Part model, mm, in its own coordinate system. A direction names the side the tool comes from. Coordinates: 2 decimals unless noted, no trailing zeros. Loops run counter-clockwise (first coordinate to the right, second up) from the corner with the lowest first, then second, coordinate; pieces in that order, holes last. Notation, with made-up numbers: M -38,-1 L -13,-1 A18 ccw -13,10 Z; hole C -8,70.5 d9. An arc over 180 degrees is marked long. Answer as a JSON object with one key per item and string values. Group by question number.
1. Saw through at C-C on z = 59. Write the cut outline in (x, y), then the cut area to 3 significant figures.
2. 3-axis set-ups, long thin cutter, end or side, ignore diameter. For faces 1 (the face through (-2, 6, 0)), 2 (the face through (-1.73, -7.81, 241.57)), 3 (the face through (-4, 4, 497)): which of +Z, -Z, +X, -X, +Y, -Y reach the whole face in a straight line?
3. Drill centre lines: L1, parallel to Z at x = -4.25, y = 5.75; L2, parallel to Y at x = 1.25, z = 266.5; L3, parallel to Z at x = 3.5, y = 3.5. Where is each one in solid material? Low to high.
4. Drop flat-ended pins along their axis: pin 1 Ø1 at (x, z) = (2.5, 115) entering from +Y; pin 2 Ø1 at (x, z) = (4, 143.5) entering from +Y; pin 3 Ø5 at (y, z) = (-5, 69) entering from +X. Give the stop position or say it passes through.
from build123d import *

# Parameters (mm, degrees)
SKETCH1_R           = 8
BOSS_EXTRUDE1_DEPTH = 490
SKETCH6_R           = 6
BOSS_EXTRUDE2_DEPTH = 5
SKETCH7_R           = 6
BOSS_EXTRUDE3_DEPTH = 2
SKETCH8_R           = 5
BOSS_EXTRUDE4_DEPTH = 10
SKETCH9_R           = 4
BOSS_EXTRUDE5_DEPTH = 10
CHAMFER1_SIZE       = 1
CHAMFER2_SIZE       = 1
BOSS_EXTRUDE6_START = 5
SKETCH10_R          = 6
BOSS_EXTRUDE6_DEPTH = 5
BOSS_EXTRUDE7_START = 2
SKETCH11_R          = 6
BOSS_EXTRUDE7_DEPTH = 2
BOSS_EXTRUDE8_START = 10
SKETCH12_R          = 5
BOSS_EXTRUDE8_DEPTH = 10
CHAMFER3_SIZE       = 1


with BuildPart() as part:
    # Sketch1 → Boss-Extrude1 (new body)
    with BuildSketch(Plane.XY):
        Circle(SKETCH1_R)
    extrude(amount=BOSS_EXTRUDE1_DEPTH)

    # Sketch6 → Boss-Extrude2 (add)
    with BuildSketch(Plane(origin=(0, 0, 0), x_dir=(-1, 0, 0), z_dir=(0, 0, -1))):
        with Locations(Location((0, 0, 0), (0, 0, 180))):
            Circle(SKETCH6_R)
    extrude(amount=BOSS_EXTRUDE2_DEPTH)

    # Sketch7 → Boss-Extrude3 (add)
    with BuildSketch(Plane(origin=(0, 0, -5), x_dir=(-1, 0, 0), z_dir=(0, 0, -1))):
        with Locations(Location((0, 0, 0), (0, 0, 180))):
            Circle(SKETCH7_R)
    extrude(amount=BOSS_EXTRUDE3_DEPTH)

    # Sketch8 → Boss-Extrude4 (add)
    with BuildSketch(Plane(origin=(0, 0, -7), x_dir=(-1, 0, 0), z_dir=(0, 0, -1))):
        Circle(SKETCH8_R)
    extrude(amount=BOSS_EXTRUDE4_DEPTH)

    # Sketch9 → Boss-Extrude5 (add)
    with BuildSketch(Plane(origin=(0, 0, -17), x_dir=(-1, 0, 0), z_dir=(0, 0, -1))):
        Circle(SKETCH9_R)
    extrude(amount=BOSS_EXTRUDE5_DEPTH)

    # Chamfer1
    chamfer1_edges = [part.edges().sort_by_distance(p)[0] for p in [
        (5, 0, -17),
    ]]
    chamfer(chamfer1_edges, length=CHAMFER1_SIZE - 0.0001)  # a hair under: the kernel refuses the full size

    # Chamfer2
    chamfer2_edges = [part.edges().sort_by_distance(p)[0] for p in [
        (4, 0, -27),
    ]]
    chamfer(chamfer2_edges, length=CHAMFER2_SIZE)

    # Sketch10 → Boss-Extrude6 (add)
    with BuildSketch(Plane.XY.offset(490).offset(BOSS_EXTRUDE6_START)):
        Circle(SKETCH10_R)
    extrude(amount=-BOSS_EXTRUDE6_DEPTH)

    # Sketch11 → Boss-Extrude7 (add)
    with BuildSketch(Plane.XY.offset(495).offset(BOSS_EXTRUDE7_START)):
        Circle(SKETCH11_R)
    extrude(amount=-BOSS_EXTRUDE7_DEPTH)

    # Sketch12 → Boss-Extrude8 (add)
    with BuildSketch(Plane.XY.offset(497).offset(BOSS_EXTRUDE8_START)):
        with Locations(Location((0, 0, 0), (0, 0, 180))):
            Circle(SKETCH12_R)
    extrude(amount=-BOSS_EXTRUDE8_DEPTH)

    # Chamfer3
    chamfer3_edges = [part.edges().sort_by_distance(p)[0] for p in [
        (5, 0, 507),
    ]]
    chamfer(chamfer3_edges, length=CHAMFER3_SIZE)


solid = part.part
Outcome:
{
 "1": {"outline": "C 0,0 d16", "area": "201 mm²"},
 "2": {"face 1": "-Z", "face 2": "+Z, -Z", "face 3": "+Z"},
 "3": {"L1": "z = 0 to 490", "L2": "y = -7.9 to 7.9", "L3": "z = -16.05 to 506.05"},
 "4": {"pin 1": "stops at y = 7.75", "pin 2": "stops at y = 7.19", "pin 3": "stops at x = 7.6"}
}
